Here's the drawing with two shaded views (mm, measured from the low corner). I have some questions. A direction names the side the tool comes from. Round coordinates to 2 decimals unless told otherwise and drop trailing zeros. Order: outer loops, then holes, each group sorted by start corner. A loop starts at its lowest first (then second) coordinate and runs counter-clockwise, first axis right, second up.
Q1. We'd pull the mould along X, two halves only. Please class the marked faces 1, 2 and 3: pulls with the +X half, pulls with the -X half, needs draft (parallel to the pull), parting line crosses it, or undercut.
Q2. If we section it at C-C (y = 23.5): Please give me the cut outline in (x, z), plus the area to 3 significant figures.
Q3. If we section it at D-D (z = 37): Please give me the cut outline in (x, y).
Q4. If we section it at B-B (y = 7.8): Please give me the cut outline in (x, z).
Q5. If we section it at A-A (z = 31.9): Please give me the cut outline in (x, y), plus the area to 3 significant figures.
Q6. For the marked faces 4, 5 and 6, which set-ups out of +Z, -Z, +X, -X, +Y, -Y let a thin tool reach every point of the face, with its end or its side?
Q7. Will these pins go through, and if not, where does the flat tip stop? P1, Ø2.5, axis at x = 3, y = 27.5, coming from the -Z side; P2, Ø6, axis at x = 36.5, y = 15, coming from the +Z side; P3, Ø1.5, axis at x = 18.5, z = 24, coming from the +Y side; P4, Ø5.5, axis at x = 41.5, z = 17, coming from the +Y side.
Q8. If I drill on line 1 (Y direction, x = 3, z = 37); line 2 (X direction, y = 5.5, z = 5); line 3 (Z direction, x = 40.5, y = 7.8), over which ranges is the centre line in solid material (lowest first)?
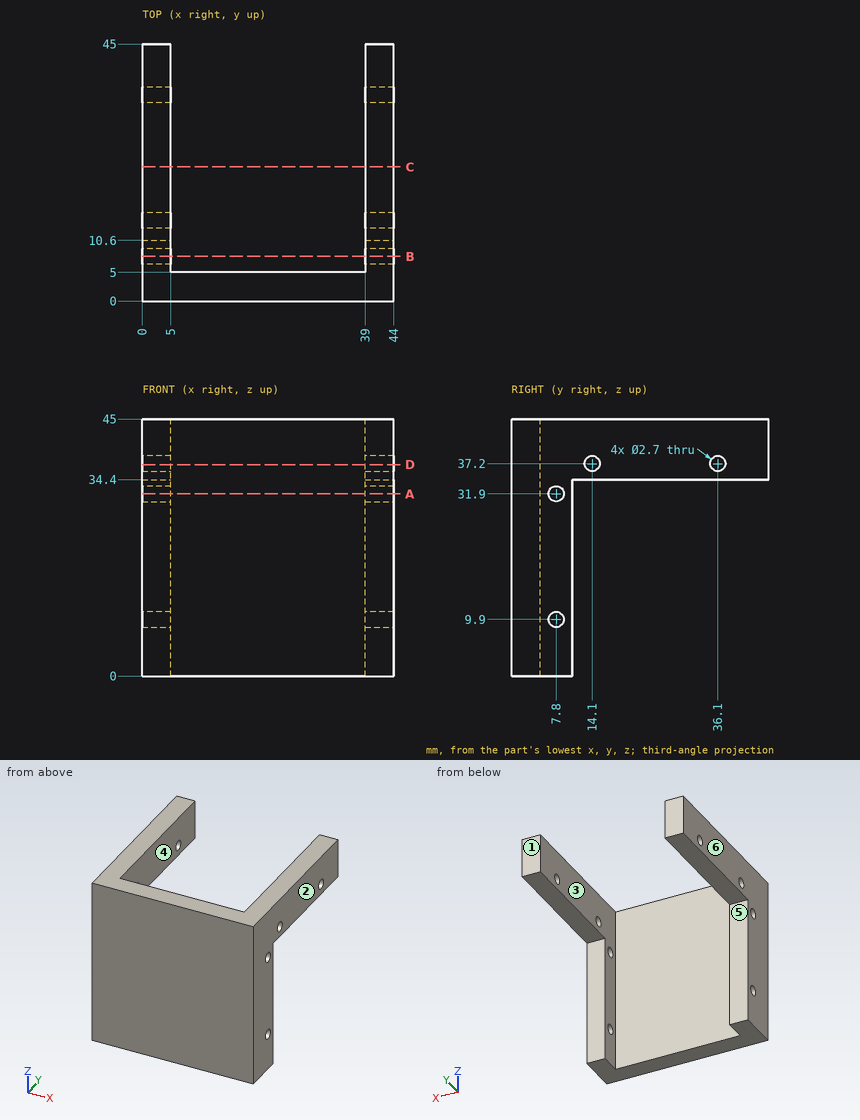
Solution:
1. face 1: needs draft
1. face 2: pulls with the +X half
1. face 3: undercut
2. outline: (0, 34.4) - (5, 34.4) - (5, 45) - (0, 45) - close; (39, 34.4) - (44, 34.4) - (44, 45) - (39, 45) - close
2. area: 106 mm2
3. outline: (0, 0) - (44, 0) - (44, 12.76) - (39, 12.76) - (39, 5) - (5, 5) - (5, 12.76) - (0, 12.76) - close; (0, 15.44) - (5, 15.44) - (5, 34.76) - (0, 34.76) - close; (0, 37.44) - (5, 37.44) - (5, 45) - (0, 45) - close; (39, 15.44) - (44, 15.44) - (44, 34.76) - (39, 34.76) - close; (39, 37.44) - (44, 37.44) - (44, 45) - (39, 45) - close
4. outline: (0, 0) - (5, 0) - (5, 8.55) - (0, 8.55) - close; (0, 11.25) - (5, 11.25) - (5, 30.55) - (0, 30.55) - close; (0, 33.25) - (5, 33.25) - (5, 45) - (0, 45) - close; (39, 0) - (44, 0) - (44, 8.55) - (39, 8.55) - close; (39, 11.25) - (44, 11.25) - (44, 30.55) - (39, 30.55) - close; (39, 33.25) - (44, 33.25) - (44, 45) - (39, 45) - close
5. outline: (0, 0) - (44, 0) - (44, 6.45) - (39, 6.45) - (39, 5) - (5, 5) - (5, 6.45) - (0, 6.45) - close; (0, 9.15) - (5, 9.15) - (5, 10.6) - (0, 10.6) - close; (39, 9.15) - (44, 9.15) - (44, 10.6) - (39, 10.6) - close
5. area: 249 mm2
6. face 4: +Z, -Z, +Y
6. face 5: -Z, +X, -X, +Y
6. face 6: +Z, -Z, -X, +Y, -Y
7. P1: stops at z = 34.4
7. P2: stops at z = 45
7. P3: stops at y = 5
7. P4: stops at y = 10.6
8. line 1: y = 0 to 12.76, 15.44 to 34.76, 37.44 to 45
8. line 2: x = 0 to 5, 39 to 44
8. line 3: z = 0 to 8.55, 11.25 to 30.55, 33.25 to 45
